from build123d import *

# Parameters (mm, degrees)
F0_R     = 5
F1_DEPTH = 10
F3_D     = 4.2
F3_DEPTH = 14.4
F3_TIP   = 1.2618073
F5_D     = 2.5
F5_DEPTH = 8
F5_START = 0.1316528
F5_TIP   = 0.7510757738


with BuildPart() as f1:
    # F0 (on Front) → F1 (new body)
    with BuildSketch(Plane.XZ):
        with BuildLine():
            Line((8, 12.5), (-8, 12.5))
            Line((-8, 12.5), (-8, -6.5))
            ThreePointArc((-8, -6.5), (-6.2426406871, -10.7426406871), (-2, -12.5))
            Line((-2, -12.5), (2, -12.5))
            ThreePointArc((2, -12.5), (6.2426406871, -10.7426406871), (8, -6.5))
            Line((8, -6.5), (8, 12.5))
        make_face()
        with Locations((0, -4.5)):
            Circle(F0_R, mode=Mode.SUBTRACT)
    extrude(amount=-F1_DEPTH)

    # F3
    with Locations(Plane.XY.offset(12.5)):
        with Locations((-4, 5), (4, 5)):
            Hole(F3_D / 2, depth=F3_DEPTH)
            with Locations((0, 0, -(F3_DEPTH + F3_TIP / 2))):  # 118° drill point
                Cone(0, F3_D / 2, F3_TIP, mode=Mode.SUBTRACT)

    # F5
    # its depths count from where the whole tool has entered the part; down to there all is cleared
    with Locations(Plane.YZ.offset(8).offset(-F5_START)):
        with Locations((5, -6.5)):
            Hole(F5_D / 2, depth=F5_DEPTH)
            with Locations((0, 0, -(F5_DEPTH + F5_TIP / 2))):  # 118° drill point
                Cone(0, F5_D / 2, F5_TIP, mode=Mode.SUBTRACT)


solid = f1.part
Can you work these out from the model? Positions are in its coordinate system, mm. A direction names the side the tool comes from. Coordinates: 2 decimals unless noted, no trailing zeros. Loops run counter-clockwise (first coordinate to the right, second up) from the corner with the lowest first, then second, coordinate; pieces in that order, holes last. Notation, with made-up numbers: M 7.5,-33 L 23.5,-33 A17 cw 23.5,-22 Z; hole C -28,6 d5. An arc over 180 degrees is marked long. Answer as CSV lines item,"result". Start each with the question number.
1. Suppose I cut it at A-A, the plane x = 0. List the corners of the cut face in (y, z) for me.
2. If I drill on probe 1 along X at (y, z) = (5, 7.25); probe 2 along Z at (x, y) = (-0.25, 4.25); probe 3 along X at (y, z) = (4, 10.75), over which ranges is the centre line in solid material (lowest first)? Write a range as [from, to].
3. Thinking about a two-plate mould opening in X: for faces 4 (the face through (-1.08, 4.93, -9.38)), 5 (the face through (-8, 5, 3)), 6 (the face through (6.196, 4.93, -10.789)), which applies, +X half, -X half, draft (parallel to the pull), parting line (faces both ways), or undercut?
4. For pin 1 Ø3.5 at (x, y) = (-4, 5) entering from +Z; pin 2 Ø4 at (x, y) = (4, 5) entering from +Z; pin 3 Ø4 at (x, y) = (-4.5, 6) entering from -Z, each with a flat end and sliding along its axis, tell me the tip position at first contact or that it passes through.
5. For faces 1 (the face through (-5.237, 5.025, -2.418)), 2 (the face through (8, 5, 3)), 3 (the face through (6.33, 5.27, -7.72)), which set-ups out of +Z, -Z, +X, -X, +Y, -Y let a thin tool reach every point of the face, with its end or its side?
6. Suppose I cut it at B-B, the plane y = 9. List the corners of the cut face in (x, z) for me.
7. Suppose I cut it at D-D, the plane z = 8. List the corners of the cut face in (x, y) for me.
8. Suppose I cut it at C-C, the plane z = -4.5. List the corners of the cut face in (x, y) for me.
Output:
1,outline,"M 0,-12.5 L 10,-12.5 L 10,-9.5 L 0,-9.5 Z; M 0,0.5 L 10,0.5 L 10,12.5 L 0,12.5 Z"
2,probe 1,"x = [-8, -6.1], [-1.9, 1.9], [6.1, 8]"
2,probe 2,"z = [-12.5, -9.49], [0.49, 12.5]"
2,probe 3,"x = [-8, -5.85], [-2.15, 2.15], [5.85, 8]"
3,face 4,"undercut"
3,face 5,"-X half"
3,face 6,"+X half"
4,pin 1,"stops at z = -2.11"
4,pin 2,"stops at z = -1.96"
4,pin 3,"stops at z = -12.48"
5,face 1,"+Z"
5,face 2,"+Z, -Z, +X, +Y, -Y"
5,face 3,"+X"
6,outline,"M -8,-6.5 A6 ccw -2,-12.5 L 2,-12.5 A6 ccw 8,-6.5 L 8,12.5 L -8,12.5 Z; hole C 0,-4.5 d10"
7,outline,"M -8,0 L 8,0 L 8,10 L -8,10 Z; hole C -4,5 d4.2; hole C 4,5 d4.2"
8,outline,"M -8,0 L -5,0 L -5,10 L -8,10 Z; M 5,0 L 8,0 L 8,10 L 5,10 Z"
